from build123d import *

# Parameters (mm, degrees)
F1_DEPTH = 5.715
F2_R     = 1.5875
F3_DEPTH = 4.1656
F4_R     = 1.5875
F5_DEPTH = 3.81
F7_DEPTH = 5.842


with BuildPart() as f1:
    # F0 (on Top) → F1 (new body, symmetric)
    with BuildSketch(Plane.XY):
        with BuildLine():
            Line((3.5549216614, 1.5875), (0, 1.5875))
            ThreePointArc((0, 1.5875), (-1.1225320151, 1.1225320151), (-1.5875, 0))
            Line((-1.5875, 0), (-1.5875, -2.2225))
            Line((-1.5875, -2.2225), (-9.3345, -1.3589))
            Line((-9.3345, -1.3589), (-9.3345, 1.5875))
            Line((-9.3345, 1.5875), (-9.608742781, 1.5875))
            Line((-9.608742781, 1.5875), (-13.5255, -1.7653))
            Line((-13.5255, -1.7653), (-24.8539, -2.2225))
            ThreePointArc((-24.8539, -2.2225), (-26.3770597496, -3.8407239016), (-24.7898826087, -5.3962086948))
            Line((-24.7898826087, -5.3962086948), (4.7834118114, -5.3962086948))
            ThreePointArc((4.7834118114, -5.3962086948), (4.9527721319, -5.3729059822), (5.1095456268, -5.3047296971))
            ThreePointArc((5.1095456268, -5.3047296971), (6.8320364553, -3.9473788403), (8.1809379528, -2.2182632419))
            ThreePointArc((8.1809379528, -2.2182632419), (8.238795955, -2.0926103635), (8.2676969204, -1.9573294393))
            ThreePointArc((8.2676969204, -1.9573294393), (9.2733035869, 4.537554361), (10.9688257926, 10.8873547355))
            ThreePointArc((10.9688257926, 10.8873547355), (10.9628913183, 11.2928057385), (10.7101033421, 11.6098608961))
            ThreePointArc((10.7101033421, 11.6098608961), (8.8799829062, 12.3144977387), (6.9200560471, 12.2471137853))
            ThreePointArc((6.9200560471, 12.2471137853), (6.6220302078, 12.0799126553), (6.4559206195, 11.7812770521))
            Line((6.4559206195, 11.7812770521), (4.1652633995, 2.0706188245))
            ThreePointArc((4.1652633995, 2.0706188245), (3.9441262464, 1.7228965355), (3.5549216614, 1.5875))
        make_face()
    extrude(amount=F1_DEPTH, both=True)

    # F2 (on face) → F3 (join)
    with BuildSketch(Plane(origin=(0, 0, -5.715), x_dir=(1, 0, 0), z_dir=(0, 0, -1))):
        Circle(F2_R)
    extrude(amount=F3_DEPTH)

    # F4 (on face) → F5 (join)
    with BuildSketch(Plane.XY.offset(5.715)):
        Circle(F4_R)
    extrude(amount=F5_DEPTH)

    # F6 (on face) → F7 (cut)
    with BuildSketch(Plane(origin=(0, 0, -5.715), x_dir=(1, 0, 0), z_dir=(0, 0, -1))):
        with BuildLine():
            Line((9.2012649402, 17.4278523773), (0, 5.3962086948))
            ThreePointArc((0, 5.3962086948), (1.5278567181, 2.7004632752), (1.5367644299, -0.3981348225))
            ThreePointArc((1.5367644299, -0.3981348225), (0.9716267852, -1.255427274), (0, -1.5875))
            Line((0, -1.5875), (-3.6485670134, -20.050900057))
            Line((-3.6485670134, -20.050900057), (23.1213513762, -22.8752493858))
            Line((23.1213513762, -22.8752493858), (9.2012649402, 17.4278523773))
        make_face()
    extrude(amount=-F7_DEPTH, mode=Mode.SUBTRACT)

    # F8 (on Top) → F9 (revolve, cut)
    with BuildSketch(Plane.XY):
        Polygon((-9.3345, -2.3811933066), (-1.5875, -3.2447933066), (-1.5875, 2.2244379615), (-13.4883278617, 2.3323959991), (-13.5255, -1.7653), (-9.608742781, 0.5715), (-9.3345, 0.5715), align=None)
    revolve(axis=Axis((0.2309344709, 14.1097, 0), (1, 0, 0)), mode=Mode.SUBTRACT)


solid = f1.part
Model file for the job. Use its own axes, mm. A direction names the side the tool comes from. Give positions to 0.01 mm unless a question says otherwise; leave off trailing zeros. Loops run counter-clockwise (first coordinate to the right, second up) from the corner with the lowest first, then second, coordinate; pieces in that order, holes last.
1) Pull direction X, two halves, no side cores. Call faces 1 (the flat face through (-1.588, -2, 0)), 2 (the flat face through (0, 0, -9.881)), 3 (the cylindrical face through (6.81, -3.97, 2.96)), 4 (the conical face through (-5.41, -2.82, 0.08)): +X half, -X half, draft (parallel to the pull), parting line (faces both ways), or undercut.
2) Wall check: line 1 (Z direction, x = 7.5, y = 7) (3 decimals); line 2 (X direction, y = -0.5, z = -1.25); line 3 (X direction, y = -1.25, z = 4.75). Give the ranges that are in metal, low to high.
3) Saw through at B-B (x = -13). Write the cut outline in (y, z) (3 decimals).
4) Saw through at C-C (y = 3.25). Write the cut outline in (x, z) (3 decimals), plus the area to 3 significant figures.
5) Saw through at D-D (x = -7.5). Write the cut outline in (y, z) (3 decimals).
6) Tool access for faces 5 (the cylindrical face through (8.91, 12.31, 2.96)), 6 (the cylindrical face through (1.516, -2.743, -2.835)), 7 (the flat face through (-9.334, 0, 0)), 8 (the flat face through (2, 1.588, 3)): list every direction of +Z, -Z, +X, -X, +Y, -Y with a clear straight run to the whole face (end or side of a thin tool).
7) Saw through at A-A (z = -7.25). Write the cut outline in (x, y) (1 decimal), plus the area to 3 significant figures.
8) Flat gauge pins, fed straight in: pin 1 Ø2 at (x, z) = (1.5, 4.5) entering from +Y; pin 2 Ø5 at (y, z) = (3.5, -6) entering from +X; pin 3 Ø1 at (y, z) = (-2, 0.5) entering from -X. Where does each tip first touch, or does it go through?
Answer block:
1. face 1: undercut
1. face 2: draft
1. face 3: +X half
1. face 4: undercut
2. line 1: z = 0.127 to 5.715
2. line 2: x = -11.49 to -9.33, -1.59 to 1.7
2. line 3: x = -12.92 to -9.33, -1.59 to 8.34
3. outline: (-5.396, -5.715) - (-1.315, -5.715) - (-1.315, -2.055) arc R15.561 cw to (-1.315, 2.055) - (-1.315, 5.715) - (-5.396, 5.715) - close
4. outline: (4.443, 0.127) - (9.017, 0.127) - (9.017, 5.715) - (4.443, 5.715) - close
4. area: 25.6 mm2
5. outline: (-5.396, -5.715) - (-1.577, -5.715) arc R16.695 cw to (-1.577, 5.715) - (-5.396, 5.715) - close
6. face 5: +Z, -Z, +Y
6. face 6: -Z, +X
6. face 7: +Y
6. face 8: +Z, -Z, -X, +Y
7. outline: circle Ø3.2 at (0, 0)
7. area: 7.92 mm2
8. pin 1: stops at y = 1.59
8. pin 2: stops at x = 1.23
8. pin 3: stops at x = -25.69
